The model under review builds one solid part; all positions refer to its coordinate system, in mm. A direction names the side the tool comes from. Coordinates: 2 decimals unless noted, no trailing zeros. Write each loop counter-clockwise with the first axis right and the second up, starting at its lowest first coordinate (ties: lowest second). Pieces come first, ordered by that corner, then holes. Notation, with made-up numbers: (48, 70) -> (100, 70) arc R20 ccw to (100, 103) -> close; hole circle Ø2 at (16, 59). An arc over 180 degrees is marked (long way). Put each result on its own line as item: value. Start each with the question number.
from build123d import *

# Parameters (mm, degrees)
BROCA_DE_ROSQUEAR_PARA_TARRAXA_DE_M2_2X0_REACH = 32.887
BROCA_DE_ROSQUEAR_PARA_TARRAXA_DE_M2_2_R       = 0.875


with BuildPart() as part:
    # Esboço3 → Revolução1 (revolve)
    with BuildSketch(Plane.XY, mode=Mode.PRIVATE) as revolu_o1_sk:
        Polygon((0, 17), (0, 2), (-18, 2), (-18, 5), (-8, 5), (-8, 17), align=None)
    revolve(revolu_o1_sk.sketch.rotate(Axis((0, 0, 0), (-1, 0, 0)), 90), axis=Axis((0, 0, 0), (-1, 0, 0)))

    # Broca de rosquear para tarraxa de M2 2 (on position points) → Broca de rosquear para tarraxa de M2.2x0.451 (cut, up to next)
    with BuildSketch(Plane(origin=(-13.453220178, 5, 0), x_dir=(0, 0, 1), z_dir=(0, 1, 0)), mode=Mode.PRIVATE) as broca_de_rosquear_para_tarraxa_de_m2_2x0_sk1:
        Circle(BROCA_DE_ROSQUEAR_PARA_TARRAXA_DE_M2_2_R)
    broca_de_rosquear_para_tarraxa_de_m2_2x0_tool1 = extrude(broca_de_rosquear_para_tarraxa_de_m2_2x0_sk1.sketch, amount=-BROCA_DE_ROSQUEAR_PARA_TARRAXA_DE_M2_2X0_REACH, mode=Mode.PRIVATE) & part.part
    add(broca_de_rosquear_para_tarraxa_de_m2_2x0_tool1.solids().sort_by_distance((-13.45322, 5, 0))[0], mode=Mode.SUBTRACT)


solid = part.part
1. Consider section C-C on x = -5. State the section outline as (y, z) points.
2. Tool access review of faces 1 (the cylindrical face through (-13, 0, 5)), 2 (the flat face through (0, 0, -4)), 3 (the cylindrical face through (-14.23, 3.42, 0.4)): name each direction out of +Z, -Z, +X, -X, +Y, -Y from which nothing blocks a thin tool from reaching the whole face with its end or side.
3. Consider section D-D on z = -14. State the section outline as (x, y) points.
4. Insertion check: P1, Ø6, axis at y = -5.5, z = 8.5, coming from the +X side; P2, Ø1.5, axis at y = 1, z = -9.5, coming from the -X side; P3, Ø2.5, axis at x = -13.45, z = 0, coming from the +Y side; P4, Ø1.5, axis at x = -8.5, z = -3, coming from the +Y side. Each pin has a flat end and moves straight along its axis. Give the tip position at first contact, or say it passes through.
5. The part is to be moulded in two halves that separate along Z. For faces 4 (the cylindrical face through (-9.126, -1.686, -1.075)), 5 (the flat face through (-8, 4, 4)), 6 (the cylindrical face through (-3.944, -16.855, 2.213)), say which applies: released by +Z, released by -Z, zero draft, split by the parting line, or undercut.
6. Consider section B-B on y = 0. State the section outline as (x, z) points.
7. Consider section A-A on z = 0. State the section outline as (x, y) points, then the cut area to 3 significant figures.
8. Wall thickness on line 1 (X direction, y = 4, z = 0); line 2 (Y direction, x = -12.25, z = 0); line 3 (Y direction, x = -5, z = 0): over which ranges is each line inside the solid? List them lowest first. Write a range as from..to.
Output values:
1. outline: circle Ø34 at (0, 0); hole circle Ø4 at (0, 0)
2. face 1: -X
2. face 2: +Z, -Z, +X, +Y, -Y
2. face 3: +Y
3. outline: (-8, -9.64) -> (0, -9.64) -> (0, 9.64) -> (-8, 9.64) -> close
4. P1: stops at x = 0
4. P2: stops at x = -8
4. P3: stops at y = 5
4. P4: stops at y = 16.82
5. face 4: undercut
5. face 5: zero draft
5. face 6: split by the parting line
6. outline: (-18, -5) -> (-8, -5) -> (-8, -17) -> (0, -17) -> (0, -2) -> (-18, -2) -> close; (-18, 2) -> (0, 2) -> (0, 17) -> (-8, 17) -> (-8, 5) -> (-18, 5) -> close
7. outline: (-18, -5) -> (-8, -5) -> (-8, -17) -> (0, -17) -> (0, -2) -> (-18, -2) -> close; (-18, 2) -> (-14.33, 2) -> (-14.33, 5) -> (-18, 5) -> close; (-12.58, 2) -> (0, 2) -> (0, 17) -> (-8, 17) -> (-8, 5) -> (-12.58, 5) -> close
7. area: 295 mm^2
8. line 1: x = -18..-14.33, -12.58..0
8. line 2: y = -5..-2, 2..5
8. line 3: y = -17..-2, 2..17
